Verification items for the finished model (mm, model axes). A direction names the side the tool comes from. Give positions to 0.01 mm unless a question says otherwise; leave off trailing zeros. Write each loop counter-clockwise with the first axis right and the second up, starting at its lowest first coordinate (ties: lowest second). Pieces come first, ordered by that corner, then holes.
from build123d import *

# Parameters (mm, degrees)
F0_R      = 5
F1_DEPTH  = 12
F0_R_2    = 5.3391988331
F2_DEPTH  = 12
F3_DEPTH  = 6
F4_DEPTH  = 1
F0_R_3    = 8
F0_R_4    = 6
F5_DEPTH  = 1
F8_DEPTH  = 10
F9_SIZE2  = 5
F9_SIZE   = 2
F10_DEPTH = 2


with BuildPart() as f1:
    # F0 (on Top) → F1 (new body)
    with BuildSketch(Plane.XY):
        Circle(F0_R)
    extrude(amount=F1_DEPTH)

    # F0 (on Top) → F2 (join)
    with BuildSketch(Plane.XY):
        Circle(F0_R_2)
        Circle(F0_R, mode=Mode.SUBTRACT)
    extrude(amount=F2_DEPTH)

    # F0 (on Top) → F3 (cut)
    with BuildSketch(Plane.XY):
        Circle(F0_R_2)
        Circle(F0_R, mode=Mode.SUBTRACT)
    extrude(amount=F3_DEPTH, mode=Mode.SUBTRACT)

    # F0 (on Top) → F4 (join)
    with BuildSketch(Plane.XY):
        Circle(F0_R_2)
        Circle(F0_R, mode=Mode.SUBTRACT)
    extrude(amount=F4_DEPTH)



with BuildPart() as f4:
    # F0 (on Top) → F4, piece 2 (new body)
    with BuildSketch(Plane.XY):
        Circle(F0_R_3)
        Circle(F0_R_4, mode=Mode.SUBTRACT)
    extrude(amount=F4_DEPTH)


with BuildPart() as f1_1:
    add(f1.part)

    add(f4.part)  # F5 merges F4
    # F0 (on Top) → F5 (join)
    with BuildSketch(Plane.XY):
        Circle(F0_R_4)
        Circle(F0_R_2, mode=Mode.SUBTRACT)
    extrude(amount=F5_DEPTH)

    # F7 (on offset) → F8 (cut)
    with BuildSketch(Plane.XY.offset(12.5)):
        Polygon((-0.5972407078, -6.0852188617), (0.5972407078, -6.0852188617), (0.5972407078, -0.5560389838), (5.559894722, -0.5560389838), (5.559894722, 0.5560389838), (0.5972407078, 0.5560389838), (0.5972407078, 6.0852188617), (-0.5972407078, 6.0852188617), (-0.5972407078, 0.5560389838), (-5.559894722, 0.5560389838), (-5.559894722, -0.5560389838), (-0.5972407078, -0.5560389838), align=None)
    extrude(amount=-F8_DEPTH, mode=Mode.SUBTRACT)

    # F9
    f9_edges = [f1_1.edges().sort_by_distance(p)[0] for p in [
        (3.790008, -3.760703, 12),
        (-3.790008, -3.760703, 12),
        (3.790008, 3.760703, 12),
        (-3.790008, 3.760703, 12),
    ]]
    chamfer(f9_edges, length=F9_SIZE, length2=F9_SIZE2)

    # F0 (on Top) → F10 (join)
    with BuildSketch(Plane.XY):
        Circle(F0_R_3)
        Circle(F0_R_4, mode=Mode.SUBTRACT)
        Circle(F0_R_4)
        Circle(F0_R_2, mode=Mode.SUBTRACT)
        Circle(F0_R_2)
        Circle(F0_R, mode=Mode.SUBTRACT)
        Circle(F0_R)
    extrude(amount=-F10_DEPTH)


solid = f1_1.part
Item 1: Set-up check for faces 4 (the face through (0.597, 2, 7)), 5 (the face through (-2, 0.556, 7)), 6 (the face through (-3.7, -3.6, 6)), 7 (the face through (-3.83, -3.72, 6.49)): record each of +Z, -Z, +X, -X, +Y, -Y from which the full face is reachable in a straight line by a thin tool's end or side.
Answer key:
face 4: +Z, +Y, -Y
face 5: +Z, +X, -X
face 6: -X, -Y
face 7: +Z, -X, -Y
Item 2: Sectioned sample at B-B on x = 0. Record the cut outline in (y, z).
Answer key:
outline: (-8, -2) - (8, -2) - (8, 1) - (5, 1) - (5, 2.5) - (-5, 2.5) - (-5, 1) - (-8, 1) - close
Item 3: Sectioned sample at D-D on y = 6. Record the cut outline in (x, z), then the cut area to 3 significant figures.
Answer key:
outline: (-5.29, -2) - (5.29, -2) - (5.29, 1) - (-5.29, 1) - close
area: 31.7 mm2
Item 4: Scan lines: line 1 along Z through (x, y) = (-5.25, -4.5); line 2 along Z through (x, y) = (0.5, 2.5); line 3 along Y through (x, z) = (2.5, 6.5). Record each from-to range of solid material in increasing order.
Answer key:
line 1: z = -2 to 1
line 2: z = -2 to 2.5
line 3: y = -4.72 to -0.56, 0.56 to 4.72
Item 5: Release check for a two-part mould opening along Z. For faces 1 (the face through (-0.597, -2, 7)), 2 (the face through (3.12, 3.04, 9.46)), 3 (the face through (-3.7, 3.6, 6)) record: released by +Z, released by -Z, zero draft, split by the parting line, or undercut.
Answer key:
face 1: zero draft
face 2: released by +Z
face 3: undercut
Item 6: Sectioned sample at A-A on z = 8. Record the cut outline in (x, y), then the cut area to 3 significant figures.
Answer key:
outline: (-4.91, -0.56) arc R4.94 ccw to (-0.6, -4.9) - (-0.6, -0.56) - close; (-4.91, 0.56) - (-0.6, 0.56) - (-0.6, 4.9) arc R4.94 ccw to start; (0.6, -4.9) arc R4.94 ccw to (4.91, -0.56) - (0.6, -0.56) - close; (0.6, 0.56) - (4.91, 0.56) arc R4.94 ccw to (0.6, 4.9) - close
area: 55.2 mm2
Item 7: Depth check by flat-ended pin: pin 1 (1.4 mm diameter, centred on x = -2, z = 7, fed in from -Y); pin 2 (4 mm diameter, centred on y = 6.5, z = 0, fed in from +X); pin 3 (1 mm diameter, centred on y = 1, z = 8.5, fed in from +X). Enter the tip coordinate at first touch or a pass-through.
Answer key:
pin 1: stops at y = -5.18
pin 2: stops at x = 6.61
pin 3: stops at x = 4.86
